Source: three-view drawing plus pictorial views. Frame: mm from the lowest corner of the part. Coordinates: 2 decimals unless noted, no trailing zeros. Write each loop counter-clockwise with the first axis right and the second up, starting at its lowest first coordinate (ties: lowest second). Pieces come first, ordered by that corner, then holes. Notation, with made-up numbers: (65, 29) - (95, 29) arc R29 ccw to (95, 49) - close; hole circle Ø6 at (-34.75, 85.5). An arc over 180 degrees is marked (long way). Put each result on its own line as item: value. Start each with the question number.
1. Cut plane A-A, the plane x = 91.25. Return loops of the section in (y, z), and give its area (3 significant figures).
2. Cut plane B-B, the plane x = 34.5. Return loops of the section in (y, z), and give its area (3 significant figures).
3. Cut plane C-C, the plane y = 11. Count the separate pieces of the cut face and the enclosed holes in it, and give its area (3 significant figures).
4. Line query: line 1 (Y direction, x = 74, z = 1.5); line 2 (Y direction, x = 91.25, z = 0.65); line 3 (X direction, y = 8, z = 1.15) (3 decimals). Output: solid intervals per line, ascending.
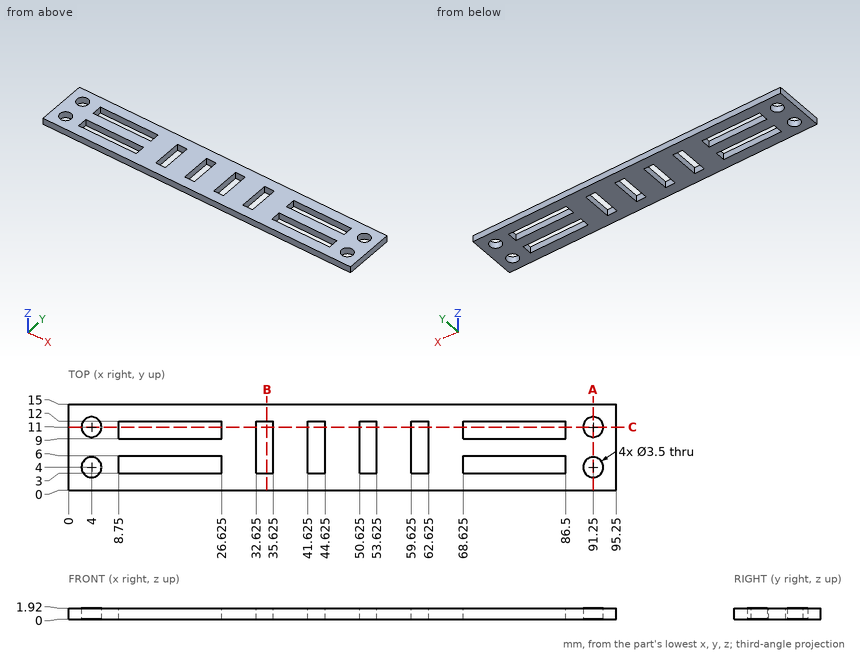
Report:
1. outline: (0, 0) - (2.25, 0) - (2.25, 1.92) - (0, 1.92) - close; (5.75, 0) - (9.25, 0) - (9.25, 1.92) - (5.75, 1.92) - close; (12.75, 0) - (15, 0) - (15, 1.92) - (12.75, 1.92) - close
1. area: 15.4 mm^2
2. outline: (0, 0) - (3, 0) - (3, 1.92) - (0, 1.92) - close; (12, 0) - (15, 0) - (15, 1.92) - (12, 1.92) - close
2. area: 11.5 mm^2
3. separate pieces: 9
3. enclosed holes: 0
3. area: 77.8 mm^2
4. line 1: y = 0 to 3, 6 to 9, 12 to 15
4. line 2: y = 0 to 2.25, 5.75 to 9.25, 12.75 to 15
4. line 3: x = 0 to 32.625, 35.625 to 41.625, 44.625 to 50.625, 53.625 to 59.625, 62.625 to 95.25
